Here's how the part is built. I have some questions about the finished solid (model axes, mm). A direction names the side the tool comes from. Round coordinates to 2 decimals unless told otherwise and drop trailing zeros. Write each loop counter-clockwise with the first axis right and the second up, starting at its lowest first coordinate (ties: lowest second). Pieces come first, ordered by that corner, then holes. Notation, with made-up numbers: (3.5, 6) - (13.5, 6) arc R15 cw to (13.5, 35) - close; hole circle Ø10 at (-1.75, 65). An arc over 180 degrees is marked (long way). Use one line per item in the form item = value. Start each with the question number.
1. I want a section at A-A, the plane x = -8.25. List the corners of the cut face in (y, z) for me, plus the area to 4 significant figures.
2. Which directions (+Z, -Z, +X, -X, +Y, -Y) give clear straight access to the entire face, cutting with the end or side of a thin tool? Please do faces 1 (the flat face through (0, 96, -3)), 2 (the flat face through (-7, 187, -1)).
3. I want a section at B-B, the plane z = -1.6. List the corners of the cut face in (x, y) for me (3 decimals), plus the area to 3 significant figures.
4. I want a section at C-C, the plane y = 96.5. List the corners of the cut face in (x, z) for me, plus the area to 4 significant figures.
5. If I drill on line 1 along Y through (x, z) = (-6.5, -1); line 2 along X through (y, z) = (43, -0.2); line 3 along X through (y, z) = (91, -0.3), over which ranges is the centre line in solid material (lowest first)?
```python
from build123d import *

# Parameters (mm, degrees)
BOSS_EXTRUDE1_DEPTH   = 195
CORTAR_EXTRUIR4_DEPTH = 10


with BuildPart() as part:
    # Sketch1 → Boss-Extrude1 (new body)
    with BuildSketch(Plane(origin=(0, 0, 0), x_dir=(1, 0, 0), z_dir=(0, 1, 0))):
        Polygon((-12.850649351, 0), (8.649350649, 0), (12.149350649, 3), (-12.850649351, 3), align=None)
    extrude(amount=BOSS_EXTRUDE1_DEPTH)

    # Croquis1 → Cortar-Extruir4 (cut)
    with BuildSketch(Plane.XY):
        with BuildLine():
            Line((-1.350649351, 4.75), (-12.850649351, 4.75))
            Line((-12.850649351, 4.75), (-12.850649351, 8))
            Line((-12.850649351, 8), (-1.350649351, 8))
            ThreePointArc((-1.350649351, 8), (0.274350649, 6.375), (-1.350649351, 4.75))
        make_face()
        with BuildLine():
            Line((-12.850649351, 187), (-1.350649351, 187))
            ThreePointArc((-1.350649351, 187), (0.274350649, 188.625), (-1.350649351, 190.25))
            Line((-1.350649351, 190.25), (-12.850649351, 190.25))
            Line((-12.850649351, 190.25), (-12.850649351, 187))
        make_face()
    extrude(amount=-CORTAR_EXTRUIR4_DEPTH, mode=Mode.SUBTRACT)


solid = part.part
```
Model answer:
q1.outline = (0, -3) - (4.75, -3) - (4.75, 0) - (0, 0) - close; (8, -3) - (187, -3) - (187, 0) - (8, 0) - close; (190.25, -3) - (195, -3) - (195, 0) - (190.25, 0) - close
q1.area = 565.5 mm2
q2.face_1 = -Z, +X, -X, +Y, -Y
q2.face_2 = +Z, -Z, -X
q3.outline = (-12.851, 0) - (10.516, 0) - (10.516, 195) - (-12.851, 195) - (-12.851, 190.25) - (-1.351, 190.25) arc R1.625 cw to (-1.351, 187) - (-12.851, 187) - (-12.851, 8) - (-1.351, 8) arc R1.625 cw to (-1.351, 4.75) - (-12.851, 4.75) - close
q3.area = 4,470 mm2
q4.outline = (-12.85, -3) - (12.15, -3) - (8.65, 0) - (-12.85, 0) - close
q4.area = 69.75 mm2
q5.line_1 = 0 to 4.75, 8 to 187, 190.25 to 195
q5.line_2 = -12.85 to 8.88
q5.line_3 = -12.85 to 9
